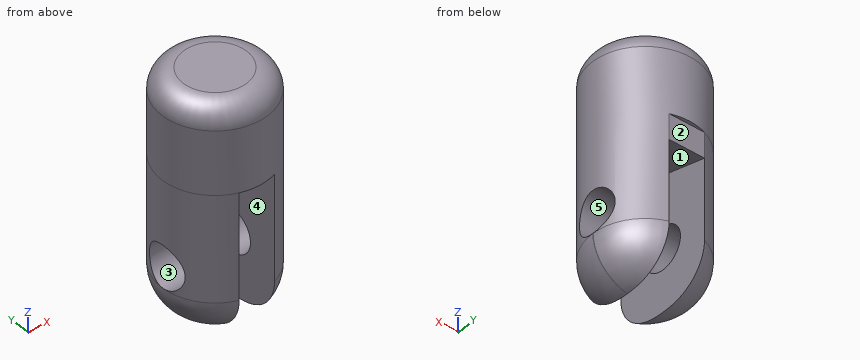
```python
from build123d import *
from build123d.topology import SkipClean

# Parameters (mm, degrees)
ESQUISSE1_R                  = 2.5
BOSS_EXTRU_1_DEPTH           = 4
BOSS_EXTRU_2_START           = 7
BOSS_EXTRU_2_DEPTH           = 7
ENL_V_MAT_EXTRU_2_DEPTH      = 9.153066908
ENL_V_MAT_EXTRU_2_DEPTH_BACK = 9.153066908
ESQUISSE3_R                  = 1
CONG_1_R                     = 2
BOSS_EXTRU_3_REACH           = 10.127
CONG_2_R                     = 1


# Some blends are built 0.0001 mm under size
with BuildPart() as part:
    # Esquisse1 → Boss.-Extru.1 (new body)
    with BuildSketch(Plane.XY):
        Circle(ESQUISSE1_R)
    extrude(amount=BOSS_EXTRU_1_DEPTH)

    # Esquisse2 → Boss.-Extru.2 (add)
    with SkipClean():  # the faces are left unmerged after this step: merging them gives an invalid solid
        with BuildSketch(Plane(origin=(0, 0, 0), x_dir=(-1, 0, 0), z_dir=(0, 0, -1)).offset(BOSS_EXTRU_2_START)):
            with BuildLine():
                Line((0.85, -2.351063589), (0.85, 2.351063589))
                ThreePointArc((0.85, 2.351063589), (2.5, 0), (0.85, -2.351063589))
            make_face()
            with BuildLine():
                Line((-0.85, -2.351063589), (-0.85, 2.351063589))
                ThreePointArc((-0.85, 2.351063589), (-2.5, 0), (-0.85, -2.351063589))
            make_face()
        extrude(amount=-BOSS_EXTRU_2_DEPTH)

    # Esquisse3 → Enlèv. mat.-Extru.2 (cut, two sides: drawn at the far end of the back side and taken through both)
    with SkipClean():  # the faces are left unmerged after this step: merging them gives an invalid solid
        with BuildSketch(Plane.ZY.offset(-0.85).offset(-ENL_V_MAT_EXTRU_2_DEPTH_BACK)):
            with Locations((-4, 0)):
                Circle(ESQUISSE3_R)
        extrude(amount=ENL_V_MAT_EXTRU_2_DEPTH + ENL_V_MAT_EXTRU_2_DEPTH_BACK, mode=Mode.SUBTRACT)

    # Congé1
    # the kernel refuses this fillet: 2 mm, written as the material it takes off along each edge
    with BuildSketch(Plane(origin=(0, 0, -7), x_dir=(0.9999950652018581, 0.003141587485879649, 0), z_dir=(0.003141587485879649, -0.9999950652018581, 0))) as cong_1_piece_1:
        with BuildLine():
            CenterArc((2.5 - CONG_1_R, CONG_1_R), CONG_1_R, 270, 90)
            Line((2.5 - CONG_1_R, 0), (2.5, 0))
            Line((2.5, 0), (2.5, CONG_1_R))
        make_face()
    revolve(axis=Axis((0, 0, -7), (0, 0, 1)), revolution_arc=359.64, mode=Mode.SUBTRACT)
    with BuildSketch(Plane(origin=(0, 0, -7), x_dir=(-0.9999950652018581, 0.003141587485879604, 0), z_dir=(-0.003141587485879604, -0.9999950652018581, 0))) as cong_1_piece_2:
        with BuildLine():
            CenterArc((2.5 - CONG_1_R, -CONG_1_R), CONG_1_R, 0, 90)
            Line((2.5 - CONG_1_R, 0), (2.5, 0))
            Line((2.5, 0), (2.5, -CONG_1_R))
        make_face()
    revolve(axis=Axis((0, 0, -7), (0, 0, -1)), revolution_arc=359.64, mode=Mode.SUBTRACT)

    # Esquisse4 → Boss.-Extru.3 (add, up to next)
    with BuildSketch(Plane(origin=(-0.85, 0, 0), x_dir=(0, 0, -1), z_dir=(1, 0, 0)), mode=Mode.PRIVATE) as boss_extru_3_sk1:
        Polygon((0, -2.351063589), (1.2, 2.351063589), (0, 2.351063589), align=None)
    boss_extru_3_tool1 = extrude(boss_extru_3_sk1.sketch, amount=BOSS_EXTRU_3_REACH, mode=Mode.PRIVATE) - part.part
    add(boss_extru_3_tool1.solids().sort_by_distance((-0.85, 0.783688, -0.4))[0])

    # Congé2
    cong_2_edges = [part.edges().sort_by_distance(p)[0] for p in [
        (-2.5, 0, 4),
    ]]
    fillet(cong_2_edges, radius=CONG_2_R - 0.0001)  # a hair under: the kernel refuses the full size


solid = part.part
```
Check sheet for the modelled part. Datum: model origin and axes. Units: mm. Face numbers are marked on the shaded views. A direction names the side the tool comes from. Round coordinates to 2 decimals unless told otherwise and drop trailing zeros. Order: outer loops, then holes, each group sorted by start corner. A loop starts at its lowest first (then second) coordinate and runs counter-clockwise, first axis right, second up.
1) Section check A-A (z = -3.75). Record the boundary of the cut face in (x, y), and give its area (3 significant figures).
2) Tool access check on the marked faces 1, 2 and 3. Record the directions out of +Z, -Z, +X, -X, +Y, -Y that give a thin tool (end or side, any length) a straight path to the whole face; none if there is none.
3) Scan lines: line 1 (X direction, y = 0.1, z = -2.5); line 2 (Y direction, x = -1.6, z = -4); line 3 (Y direction, x = -1.25, z = -4). Record each from-to range of solid material in increasing order.
4) Section check C-C (y = 0.5). Give the number of separate pieces and of enclosed holes in the cut face, and give its area (3 significant figures).
5) Go/stop test with flat-tipped pins: pin 1 Ø1.4 at (y, z) = (0.5, -5) entering from +X; pin 2 Ø2 at (x, z) = (1, -2) entering from -Y; pin 3 Ø1.5 at (y, z) = (-2, -3.5) entering from +X; pin 4 Ø2 at (y, z) = (1.5, 1) entering from -X. Record where each tip stops, or that it passes through.
6) Mould release check, pull along X, two halves, no side actions. Record for the marked faces 4 and 5: +X half, -X half, draft (parallel to the pull), parting line (faces both ways), or undercut.
7) Section check B-B (x = 0). Record the boundary of the cut face in (y, z).
8) Section check D-D (z = 1.5). Record the boundary of the cut face in (x, y).
Result:
1. outline: (-2.3, -0.97) arc R2.5 ccw to (-0.85, -2.35) - (-0.85, -0.97) - close; (-2.3, 0.97) - (-0.85, 0.97) - (-0.85, 2.35) arc R2.5 ccw to start; (0.85, -2.35) arc R2.5 ccw to (2.3, -0.97) - (0.85, -0.97) - close; (0.85, 0.97) - (2.3, 0.97) arc R2.5 ccw to (0.85, 2.35) - close
1. area: 5.16 mm2
2. face 1: -Z, -Y
2. face 2: -Z, +X, -X, +Y
2. face 3: +X, -X
3. line 1: x = -2.5 to -0.85, 0.85 to 2.5
3. line 2: y = -1.92 to -1, 1 to 1.92
3. line 3: y = -2.17 to -1, 1 to 2.17
4. separate pieces: 3
4. enclosed holes: 0
4. area: 35.5 mm2
5. pin 1: stops at x = 2.5
5. pin 2: stops at y = -2.35
5. pin 3: stops at x = 2.17
5. pin 4: stops at x = -2.45
6. face 4: undercut
6. face 5: draft
7. outline: (-2.5, 0) - (-2.35, 0) - (2.35, -1.2) - (2.35, 0) - (2.5, 0) - (2.5, 3) arc R1 ccw to (1.5, 4) - (-1.5, 4) arc R1 ccw to (-2.5, 3) - close
8. outline: circle Ø5 at (0, 0)
